Check sheet for the modelled part. Datum: model origin and axes. Units: mm. A direction names the side the tool comes from. Round coordinates to 2 decimals unless told otherwise and drop trailing zeros. Order: outer loops, then holes, each group sorted by start corner. A loop starts at its lowest first (then second) coordinate and runs counter-clockwise, first axis right, second up.
```python
from build123d import *

# Parameters (mm, degrees)
BOSS_EXTRUDE1_DEPTH      = 33
BOSS_EXTRUDE1_DEPTH_BACK = 33
SKETCH1_R                = 16
SKETCH1_R_2              = 11
CUT_EXTRUDE1_DEPTH       = 33
BOSS_EXTRUDE2_DEPTH      = 66
CUT_EXTRUDE4_DEPTH       = 72.18434857


with BuildPart() as part:
    # Sketch1 → Boss-Extrude1 (new, two sides: drawn at the far end of the back side and taken through both)
    with BuildSketch(Plane.XY.offset(-BOSS_EXTRUDE1_DEPTH_BACK)):
        Circle(SKETCH1_R)
        Circle(SKETCH1_R_2, mode=Mode.SUBTRACT)
    extrude(amount=BOSS_EXTRUDE1_DEPTH + BOSS_EXTRUDE1_DEPTH_BACK)

    # Sketch2 → Cut-Extrude1 (cut)
    with BuildSketch(Plane.XY.offset(33)):
        with BuildLine():
            Line((-3, 10.540195713), (-3, 13.040195713))
            Line((-3, 13.040195713), (0, 13.040195713))
            Line((0, 13.040195713), (3, 13.040195713))
            Line((3, 13.040195713), (3, 10.540195713))
            ThreePointArc((3, 10.540195713), (0, 10.958819538), (-3, 10.540195713))
        make_face()
    cut_extrude1 = extrude(amount=-CUT_EXTRUDE1_DEPTH, mode=Mode.SUBTRACT)

    # Mirror2: Cut-Extrude1 across plane
    add(cut_extrude1.mirror(Plane(origin=(0, 0, 0), x_dir=(1, 0, 0), z_dir=(0, 0, -1))), mode=Mode.SUBTRACT)

    # Sketch3 → Boss-Extrude2 (add, through all)
    with BuildSketch(Plane.XY.offset(33)):
        with BuildLine():
            Line((-3, -21.335685631), (-3, -15.716233646))
            ThreePointArc((-3, -15.716233646), (-4.63488117, -15.31397651), (-6.218441038, -14.74215015))
            Line((-6.218441038, -14.74215015), (-6.218441038, -21.335685631))
            Line((-6.218441038, -21.335685631), (-3, -21.335685631))
        make_face()
        with BuildLine():
            ThreePointArc((6.218441038, -14.74215015), (4.63488117, -15.31397651), (3, -15.716233646))
            Line((3, -15.716233646), (3, -21.335685631))
            Line((3, -21.335685631), (6.218441038, -21.335685631))
            Line((6.218441038, -21.335685631), (6.218441038, -14.74215015))
        make_face()
    extrude(amount=-BOSS_EXTRUDE2_DEPTH)

    # Sketch4 → Cut-Extrude4 (cut, through all)
    with BuildSketch(Plane.XY.offset(33)):
        Polygon((-3, -10.583005244), (-3, -16.271539673), (3, -16.271539673), (3, -15.716233646), (3, -10.583005244), align=None)
    extrude(amount=-CUT_EXTRUDE4_DEPTH, mode=Mode.SUBTRACT)


solid = part.part
```
Item 1: Sectioned sample at A-A (y = 0). Record the cut outline in (x, z).
Answer:
outline: (-16, -33) - (-11, -33) - (-11, 33) - (-16, 33) - close; (11, -33) - (16, -33) - (16, 33) - (11, 33) - close
Item 2: Sectioned sample at C-C (x = -5). Record the cut outline in (y, z), and give its area (3 significant figures).
Answer:
outline: (-21.34, -33) - (-9.8, -33) - (-9.8, 33) - (-21.34, 33) - close; (9.8, -33) - (15.2, -33) - (15.2, 33) - (9.8, 33) - close
area: 1,120 mm2
Item 3: Go/stop test with flat-tipped pins: P1, Ø5, axis at x = -11.5, z = 9, coming from the -Y side; P2, Ø3.5, axis at y = -18, z = -11.5, coming from the +X side; P3, Ø6, axis at x = 10, z = 19, coming from the +Y side; P4, Ø3, axis at x = -0.5, y = 11, coming from the -Z side. Record where each tip stops, or that it passes through.
Answer:
P1: stops at y = -13.23
P2: stops at x = 6.22
P3: stops at y = 14.39
P4: passes through
Item 4: Release check for a two-part mould opening along X. For faces 1 (the flat face through (-11, -2, 33)), 2 (the flat face through (6.218, -18, 0)), 3 (the flat face through (0, 13.04, 0)) record: released by +X, released by -X, zero draft, split by the parting line, or undercut.
Answer:
face 1: zero draft
face 2: released by +X
face 3: undercut
Item 5: Access from +Z, -Z, +X, -X, +Y, -Y to the whole of each face (thin tool, end or side, straight path). Record for faces 4 (the flat face through (3, -16, 0)), 5 (the flat face through (-11, -2, -33)), 6 (the flat face through (-5, -21.336, 0)), 7 (the flat face through (-6.218, -18, 0)), 8 (the cylindrical face through (-11, 0, 0)).
Answer:
face 4: +Z, -Z, -Y
face 5: -Z, +X, -X, +Y, -Y
face 6: +Z, -Z, +X, -X, -Y
face 7: +Z, -Z, -X, -Y
face 8: +Z, -Z
Item 6: Sectioned sample at B-B (z = 5.5). Record the cut outline in (x, y), and give its area (3 significant figures).
Answer:
outline: (-6.22, -21.34) - (-3, -21.34) - (-3, -10.58) arc R11 cw to (-3, 10.58) - (-3, 13.04) - (3, 13.04) - (3, 10.58) arc R11 cw to (3, -10.58) - (3, -21.34) - (6.22, -21.34) - (6.22, -14.74) arc R16 ccw (long way) to (-6.22, -14.74) - close
area: 420 mm2
Item 7: Scan lines: line 1 along X through (y, z) = (-19, -29); line 2 along Y through (x, z) = (-8, -27.5); line 3 along Y through (x, z) = (5.5, -25). Record each from-to range of solid material in increasing order.
Answer:
line 1: x = -6.22 to -3, 3 to 6.22
line 2: y = -13.86 to -7.55, 7.55 to 13.86
line 3: y = -21.34 to -9.53, 9.53 to 15.02
Item 8: Sectioned sample at D-D (x = 12). Record the cut outline in (y, z).
Answer:
outline: (-10.58, -33) - (10.58, -33) - (10.58, 33) - (-10.58, 33) - close
